Verification items for this drawing (mm, ordinates from the low corner). Round coordinates to 2 decimals unless told otherwise and drop trailing zeros. Order: outer loops, then holes, each group sorted by start corner. A loop starts at its lowest first (then second) coordinate and runs counter-clockwise, first axis right, second up. Notation, with made-up numbers: (18.5, 76.5) - (67.5, 76.5) arc R21 ccw to (67.5, 109.5) - close; hole circle Ø10 at (86.5, 67). An arc over 180 degrees is marked (long way). One line per question, with ' | ' between items. Start each with the question number.
Q1. Sectioned sample at B-B, the plane x = 62.5. Enter the section's corners in (y, z), then the cut area to 3 significant figures.
Q2. Sectioned sample at A-A, the plane y = 12.5. Enter the section's corners in (x, z), then the cut area to 3 significant figures.
Q3. Gauge pin test, flat end, axial feed: P1, Ø1, axis at x = 124.5, z = 46.5, coming from the -Y side. Record the tip position at first contact, or that the pin passes through.
Q4. Sectioned sample at C-C, the plane z = 35.5. Enter the section's corners in (x, y).
Q5. Material ranges on line 1 along Y through (x, z) = (79, 38.5), recorded low to high.
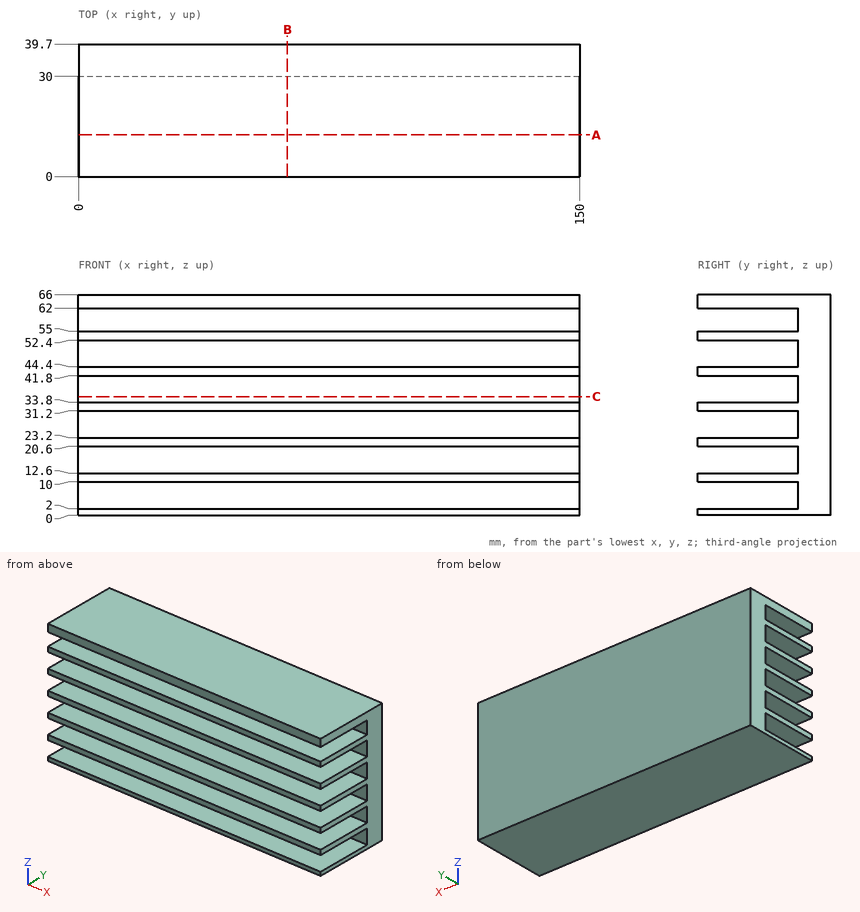
Determined:
1) outline: (0, 0) - (39.7, 0) - (39.7, 66) - (0, 66) - (0, 62) - (30, 62) - (30, 55) - (0, 55) - (0, 52.4) - (30, 52.4) - (30, 44.4) - (0, 44.4) - (0, 41.8) - (30, 41.8) - (30, 33.8) - (0, 33.8) - (0, 31.2) - (30, 31.2) - (30, 23.2) - (0, 23.2) - (0, 20.6) - (30, 20.6) - (30, 12.6) - (0, 12.6) - (0, 10) - (30, 10) - (30, 2) - (0, 2) - close | area: 1,210 mm2
2) outline: (0, 0) - (150, 0) - (150, 2) - (0, 2) - close; (0, 10) - (150, 10) - (150, 12.6) - (0, 12.6) - close; (0, 20.6) - (150, 20.6) - (150, 23.2) - (0, 23.2) - close; (0, 31.2) - (150, 31.2) - (150, 33.8) - (0, 33.8) - close; (0, 41.8) - (150, 41.8) - (150, 44.4) - (0, 44.4) - close; (0, 52.4) - (150, 52.4) - (150, 55) - (0, 55) - close; (0, 62) - (150, 62) - (150, 66) - (0, 66) - close | area: 2,850 mm2
3) P1: stops at y = 30
4) outline: (0, 30) - (150, 30) - (150, 39.7) - (0, 39.7) - close
5) line 1: y = 30 to 39.7
